Model file for the job. Use its own axes, mm. A direction names the side the tool comes from. Round coordinates to 2 decimals unless told otherwise and drop trailing zeros. Order: outer loops, then holes, each group sorted by start corner. A loop starts at its lowest first (then second) coordinate and runs counter-clockwise, first axis right, second up. Notation, with made-up numbers: (-16, -16.5) - (22, -16.5) arc R27 ccw to (22, 1.5) - close; hole circle Ø3 at (18.5, 68). An arc over 180 degrees is marked (long way). Write item = value, one per line.
```python
from build123d import *

# Parameters (mm, degrees)
SKETCH1_R           = 3.81
BOSS_EXTRUDE1_DEPTH = 77.724
SKETCH3_R           = 3.81
BOSS_EXTRUDE2_DEPTH = 6.35
SKETCH2_W           = 36.763821928
SKETCH2_H           = 29.567130372
SKETCH2_R           = 5.2451
CUT_EXTRUDE2_DEPTH  = 70.104
CUT_EXTRUDE3_START  = -1.27
SKETCH4_R           = 4.862249437
CUT_EXTRUDE3_DEPTH  = 1.27
CHAMFER1_SIZE       = 1.27
FILLET1_R           = 0.127
CHAMFER2_SIZE       = 2.54
CHAMFER2_SIZE2      = 0.680590949


with BuildPart() as part:
    # Sketch1 → Boss-Extrude1 (new body)
    with BuildSketch(Plane(origin=(0, 0, 0), x_dir=(0, 0, -1), z_dir=(1, 0, 0))):
        with BuildLine():
            Line((5.4864, -15.556063849), (-5.4864, -15.556063849))
            Line((-5.4864, -15.556063849), (-5.4864, -11.111063849))
            Line((-5.4864, -11.111063849), (-10.77595, -11.111063849))
            Line((-10.77595, -11.111063849), (-10.77595, -8.825063849))
            Line((-10.77595, -8.825063849), (-10.02746492, -8.825063849))
            Line((-10.02746492, -8.825063849), (-10.02746492, -5.434163849))
            Line((-10.02746492, -5.434163849), (-11.96975, -5.434163849))
            Line((-11.96975, -5.434163849), (-11.96975, -1.903563849))
            Line((-11.96975, -1.903563849), (-7.8867, -1.903563849))
            ThreePointArc((-7.8867, -1.903563849), (0, 5.983136151), (7.8867, -1.903563849))
            Line((7.8867, -1.903563849), (11.96975, -1.903563849))
            Line((11.96975, -1.903563849), (11.96975, -5.434163849))
            Line((11.96975, -5.434163849), (10.02746492, -5.434163849))
            Line((10.02746492, -5.434163849), (10.02746492, -8.825063849))
            Line((10.02746492, -8.825063849), (10.77595, -8.825063849))
            Line((10.77595, -8.825063849), (10.77595, -11.111063849))
            Line((10.77595, -11.111063849), (5.4864, -11.111063849))
            Line((5.4864, -11.111063849), (5.4864, -15.556063849))
        make_face()
        with Locations(Location((0, -1.903563849, 0), (0, 0, 180))):
            Circle(SKETCH1_R, mode=Mode.SUBTRACT)
    extrude(amount=BOSS_EXTRUDE1_DEPTH)

    # Sketch3 → Boss-Extrude2 (add)
    with BuildSketch(Plane(origin=(0, 0, 0), x_dir=(0, 0, -1), z_dir=(1, 0, 0))):
        with Locations(Location((0, -1.903563849, 0), (0, 0, 180))):
            Circle(SKETCH3_R)
    extrude(amount=BOSS_EXTRUDE2_DEPTH)

    # Sketch2 → Cut-Extrude2 (cut)
    with BuildSketch(Plane(origin=(0, 0, 0), x_dir=(0, 0, -1), z_dir=(1, 0, 0))):
        with Locations((-1.560728289, -3.789331886)):
            Rectangle(SKETCH2_W, SKETCH2_H)
        with Locations((0, -1.903563849)):
            Circle(SKETCH2_R, mode=Mode.SUBTRACT)
    extrude(amount=CUT_EXTRUDE2_DEPTH, mode=Mode.SUBTRACT)

    # Sketch4 → Cut-Extrude3 (cut)
    with BuildSketch(Plane(origin=(77.724, 0, 0), x_dir=(0, 0, -1), z_dir=(1, 0, 0)).offset(CUT_EXTRUDE3_START)):
        with BuildLine():
            Line((11.96975, -1.903563849), (7.8867, -1.903563849))
            ThreePointArc((7.8867, -1.903563849), (0, 5.983136151), (-7.8867, -1.903563849))
            Line((-7.8867, -1.903563849), (-11.96975, -1.903563849))
            Line((-11.96975, -1.903563849), (-11.96975, -5.434163849))
            Line((-11.96975, -5.434163849), (-10.02746492, -5.434163849))
            Line((-10.02746492, -5.434163849), (-10.02746492, -8.825063849))
            Line((-10.02746492, -8.825063849), (-10.77595, -8.825063849))
            Line((-10.77595, -8.825063849), (-10.77595, -11.111063849))
            Line((-10.77595, -11.111063849), (-5.4864, -11.111063849))
            Line((-5.4864, -11.111063849), (-5.4864, -15.556063849))
            Line((-5.4864, -15.556063849), (5.4864, -15.556063849))
            Line((5.4864, -15.556063849), (5.4864, -11.111063849))
            Line((5.4864, -11.111063849), (10.77595, -11.111063849))
            Line((10.77595, -11.111063849), (10.77595, -8.825063849))
            Line((10.77595, -8.825063849), (10.02746492, -8.825063849))
            Line((10.02746492, -8.825063849), (10.02746492, -5.434163849))
            Line((10.02746492, -5.434163849), (11.96975, -5.434163849))
            Line((11.96975, -5.434163849), (11.96975, -1.903563849))
        make_face()
        with Locations((0, -1.903563849)):
            Circle(SKETCH4_R, mode=Mode.SUBTRACT)
    extrude(amount=CUT_EXTRUDE3_DEPTH, mode=Mode.SUBTRACT)

    # Chamfer1
    # the kernel refuses this chamfer: 1.27 mm, written as the material it takes off along each edge
    with BuildSketch(Plane(origin=(77.724, -1.903563849, 0), x_dir=(0, 0, -1), z_dir=(0, -1, 0))) as chamfer1_piece_1_section:
        Polygon((4.862249437, -CHAMFER1_SIZE), (4.862249437 - CHAMFER1_SIZE, 0), (4.862249437, 0), align=None)
    chamfer1_piece_1 = revolve(axis=Axis((77.724, -1.903563849, 0), (1, 0, 0)), mode=Mode.PRIVATE)
    chamfer1_piece_1 = split(chamfer1_piece_1, bisect_by=Plane(origin=(76.454, -1.903563849, 4.22989024), z_dir=(1, 0, 0)), keep=Keep.TOP, mode=Mode.PRIVATE)
    add(chamfer1_piece_1, mode=Mode.SUBTRACT)

    # Fillet1
    fillet1_edges = [part.edges().sort_by_distance(p)[0] for p in [
        (77.506249437, 1.906436151, 0),
    ]]
    fillet(fillet1_edges, radius=FILLET1_R)

    # Chamfer2
    chamfer2_edges = [part.edges().sort_by_distance(p)[0] for p in [
        (76.454, -15.556063849, 0),
    ]]
    chamfer2_side = [part.faces().sort_by_distance(p)[0] for p in [
        (73.279, -15.556063849, 0),
    ]]
    chamfer(chamfer2_edges, length=CHAMFER2_SIZE, length2=CHAMFER2_SIZE2, reference=chamfer2_side[0])


solid = part.part
```
1) Wall check: line 1 along Y through (x, z) = (43.5, 0); line 2 along X through (y, z) = (-10.5, 7); line 3 along Z through (x, y) = (9.5, -3). Give the ranges that are in metal, low to high.
Conclusion:
line_1 = -7.15 to -5.71, 1.91 to 3.34
line_2 = 70.1 to 76.45
line_3 = -5.13 to -3.65, 3.65 to 5.13
2) Cut at B-B (z = 6.5). Write the cut outline in (x, y).
Conclusion:
outline = (70.1, -11.11) - (76.45, -11.11) - (76.45, 2.56) - (70.1, 2.56) - close
3) 3-axis set-ups, long thin cutter, end or side, ignore diameter. For faces 4 (the face through (73, -5.434, 11)), 5 (the face through (73, -10, 10.776)), 6 (the face through (70.104, -7, -2)): which of +Z, -Z, +X, -X, +Y, -Y reach the whole face in a straight line?
Conclusion:
face_4 = +Z, +X, -X
face_5 = +Z, +X, -X, -Y
face_6 = -X
4) Cut at A-A (x = 35.5). Write the cut outline in (y, z).
Conclusion:
outline = circle Ø10.49 at (-1.9, 0); hole circle Ø7.62 at (-1.9, 0)
5) Mould opens along Y. For faces 1 (the face through (73, -4, 11.97)), 2 (the face through (6.35, -2, 0)), 3 (the face through (73, -1.904, -10)) say: +Y half, -Y half, draft (parallel to the pull), parting line (faces both ways), or undercut.
Conclusion:
face_1 = draft
face_2 = undercut
face_3 = +Y half
6) Cut at C-C (z = -7). Write the cut outline in (x, y), and give its area (3 significant figures).
Conclusion:
outline = (70.1, -11.11) - (76.45, -11.11) - (76.45, 1.73) - (70.1, 1.73) - close
area = 81.5 mm^2
7) Flat gauge pins, fed straight in: pin 1 Ø1.5 at (x, y) = (49.5, -4) entering from -Z; pin 2 Ø2 at (x, z) = (74.5, -11) entering from -Y; pin 3 Ø1.3 at (x, y) = (72.5, -13.5) entering from -Z; pin 4 Ø1 at (x, y) = (60.5, -9) entering from -Z. Where does each tip first touch, or does it go through?
Conclusion:
pin_1 = -5.07
pin_2 = -11.11
pin_3 = -5.49
pin_4 = through
